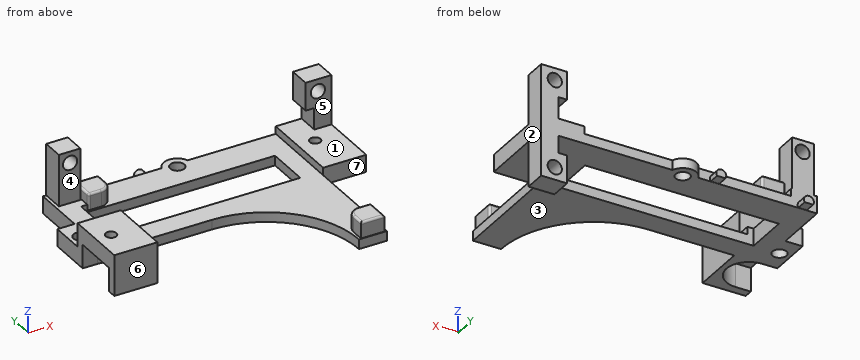
```python
from build123d import *

# Parameters (mm, degrees)
SKETCH021_R      = 1.65
EXTRUDE021_DEPTH = 5
EXTRUDE001_DEPTH = 4
FILLET003_R      = 0.5
BOX005_W         = 48
BOX005_H         = 47
BOX005_DEPTH     = 10
EXTRUDE037_DEPTH = 6
SKETCH038_W      = 10
SKETCH038_H      = 14.5
SKETCH038_R      = 1.25
EXTRUDE038_DEPTH = 4
SKETCH039_W      = 5
SKETCH039_H      = 16
SKETCH039_R      = 1.65
EXTRUDE039_DEPTH = 5
EXTRUDE040_DEPTH = 3
SKETCH020_R      = 1.65
SKETCH020_R_2    = 1.25
SKETCH020_W      = 45
SKETCH020_H      = 10
EXTRUDE036_DEPTH = 4


with BuildPart() as gpshold:
    # Sketch021 → Extrude021 (new body)
    with BuildSketch(Plane.XZ):
        Polygon((65, 28.5), (71, 28.5), (71, 2.5), (65, 2.5), (65, 9), (67, 9), (67, 22), (65, 22), align=None)
        with Locations((67.85, 25.7)):
            Circle(SKETCH021_R, mode=Mode.SUBTRACT)
        with Locations((67.85, 5.4)):
            Circle(SKETCH021_R, mode=Mode.SUBTRACT)
    extrude(amount=EXTRUDE021_DEPTH)


with BuildPart() as gpshold_1:
    # Extrude021 placement: moved
    add(gpshold.part.moved(Location((0, 78.75, 0))))


with BuildPart() as obj1:
    # Sketch001 → Extrude001 (new body)
    with BuildSketch(Plane.XY):
        with BuildLine():
            Line((19.03, 74.44), (19.03, 77.44))
            Line((19.03, 77.44), (13.53, 77.44))
            Line((13.53, 71.94), (13.53, 77.44))
            Line((16.53, 71.94), (13.53, 71.94))
            ThreePointArc((16.53, 71.94), (18.297767, 72.672233), (19.03, 74.44))
        make_face()
        with BuildLine():
            Line((60.53, 34.86), (55.03, 34.86))
            Line((55.03, 34.86), (55.03, 37.86))
            ThreePointArc((57.53, 40.36), (55.762233, 39.627767), (55.03, 37.86))
            Line((60.53, 40.36), (57.53, 40.36))
            Line((60.53, 34.86), (60.53, 40.36))
        make_face()
    extrude(amount=EXTRUDE001_DEPTH)


with BuildPart() as obj1_1:
    # Extrude001 placement: moved
    add(obj1.part.moved(Location((0, 0, 2))))

    # Fillet003
    fillet003_edges = [obj1_1.edges().sort_by_distance(p)[0] for p in [
        (57.78, 34.86, 6),
        (55.03, 36.36, 6),
        (55.762233, 39.627767, 6),
        (60.53, 40.36, 4),
        (59.03, 40.36, 6),
        (60.53, 37.61, 6),
        (18.297767, 72.672233, 6),
        (19.03, 77.44, 4),
        (19.03, 75.94, 6),
        (13.53, 77.44, 4),
        (16.28, 77.44, 6),
        (13.53, 71.94, 4),
        (13.53, 74.69, 6),
        (15.03, 71.94, 6),
    ]]
    fillet(fillet003_edges, radius=FILLET003_R)


with BuildPart() as obj1_2:
    # Fillet003 placement: moved
    add(obj1_1.part.moved(Location((0, 0, 13))))


with BuildPart() as obj2:
    # Box005 → Box005 (new body)
    with BuildSketch(Plane(origin=(13, 34, 15.25), x_dir=(1, 0, 0), z_dir=(0, 0, 1))):
        with Locations((24, 23.5)):
            Rectangle(BOX005_W, BOX005_H)
    extrude(amount=BOX005_DEPTH)


with BuildPart() as obj3:
    # Sketch037 → Extrude037 (new body)
    with BuildSketch(Plane.XY.offset(17)):
        with BuildLine():
            Line((3, 58.25), (13, 58.25))
            Line((13, 58.25), (13, 43.75))
            Line((13, 43.75), (3, 43.75))
            Line((3, 43.75), (3, 45.75))
            Line((3, 45.75), (6.5, 45.75))
            ThreePointArc((6.5, 45.75), (11.75, 51), (6.5, 56.25))
            Line((3, 56.25), (6.5, 56.25))
            Line((3, 58.25), (3, 56.25))
        make_face()
    extrude(amount=EXTRUDE037_DEPTH)


with BuildPart() as obj3_1:
    # Extrude037 placement: moved
    add(obj3.part.moved(Location((0, 0, -4))))


with BuildPart() as obj4:
    # Sketch038 → Extrude038 (new body)
    with BuildSketch(Plane.XY.offset(17)):
        with Locations((8, 51)):
            Rectangle(SKETCH038_W, SKETCH038_H)
        with Locations((6.5, 51)):
            Circle(SKETCH038_R, mode=Mode.SUBTRACT)
    extrude(amount=EXTRUDE038_DEPTH)


with BuildPart() as obj4_1:
    # Extrude038 placement: moved
    add(obj4.part.moved(Location((0, 0, 1.5))))


with BuildPart() as obj5:
    # Sketch039 → Extrude039 (new body)
    with BuildSketch(Plane.XZ.offset(-78.75)):
        with Locations((10.25, 21)):
            Rectangle(SKETCH039_W, SKETCH039_H)
        with Locations((10.35, 26.35)):
            Circle(SKETCH039_R, mode=Mode.SUBTRACT)
    extrude(amount=EXTRUDE039_DEPTH)


with BuildPart() as obj6:
    # Sketch040 → Extrude040 (new body)
    with BuildSketch(Plane.XZ.offset(-78.75)):
        with BuildLine():
            ThreePointArc((11.321071, 13.05), (10.34, 14.8), (9.358929, 13.05))
            Line((9.358929, 13.05), (11.321071, 13.05))
        make_face()
        with BuildLine():
            ThreePointArc((31.651071, 13.05), (30.67, 14.8), (29.688929, 13.05))
            Line((29.688929, 13.05), (31.651071, 13.05))
        make_face()
    extrude(amount=EXTRUDE040_DEPTH)


with BuildPart() as obj6_1:
    # Extrude040 placement: moved
    add(obj6.part.moved(Location((0, 2.5, 0))))


with BuildPart() as sensorhold005:
    # Sketch020 → Extrude036 (new body)
    with BuildSketch(Plane.XY):
        with BuildLine():
            Line((71, 78.75), (71, 60))
            Line((61, 60), (71, 60))
            Line((61, 34.75), (61, 60))
            Line((61, 34.75), (61, 60))
            Line((61, 34.75), (61, 60))
            Line((54.5, 34.75), (61, 34.75))
            ThreePointArc((54.5, 34.75), (48.202796, 49.952796), (33, 56.25))
            Line((3, 56.25), (33, 56.25))
            Line((3, 56.25), (3, 66.25))
            Line((3, 66.25), (7, 66.25))
            Line((7, 66.25), (7, 78.75))
            Line((7, 78.75), (34.55, 78.75))
            ThreePointArc((40.55, 78.75), (37.55, 80.878443), (34.55, 78.75))
            Line((40.55, 78.75), (71, 78.75))
        make_face()
        with Locations((5.55, 61.45)):
            Circle(SKETCH020_R, mode=Mode.SUBTRACT)
        with Locations((37.55, 77.7)):
            Circle(SKETCH020_R, mode=Mode.SUBTRACT)
        with Locations((65, 70)):
            Circle(SKETCH020_R_2, mode=Mode.SUBTRACT)
        with Locations((34.05, 66.45)):
            Rectangle(SKETCH020_W, SKETCH020_H, mode=Mode.SUBTRACT)
    extrude(amount=EXTRUDE036_DEPTH)


with BuildPart() as sensorhold005_1:
    # Extrude036 placement: moved
    add(sensorhold005.part.moved(Location((0, 0, 13))))

    # Fusion034: union obj3, obj4, obj5, obj6
    add(obj3_1.part)
    add(obj4_1.part)
    add(obj5.part)
    add(obj6_1.part)

    # Cut016: cut obj2
    add(obj2.part, mode=Mode.SUBTRACT)

    # Fusion035: union obj1
    add(obj1_2.part)

    # Fusion036: union gpsHold
    add(gpshold_1.part)


solid = sensorhold005_1.part
```
For this review, take the finished solid that the model builds, in its own axes (mm). Face numbers are marked on the shaded views. A direction names the side the tool comes from. Round coordinates to 2 decimals unless told otherwise and drop trailing zeros. Write each loop counter-clockwise with the first axis right and the second up, starting at its lowest first coordinate (ties: lowest second). Pieces come first, ordered by that corner, then holes. Notation, with made-up numbers: (56.5, 88.5) - (101.5, 88.5) arc R25 ccw to (101.5, 106.5) - close; hole circle Ø3 at (58.5, -20.75). An arc over 180 degrees is marked (long way). Write each question's results on one line, items separated by ' | '.
Item 1: For the marked faces 4, 5, 6 and 7, list the 3-axis set-ups (+Z, -Z, +X, -X, +Y, -Y) from which the entire face can be reached by the end or side of a thin tool; tool diameter is ignored.
Calculated:
face 4: +Z, -X | face 5: +Z, +X, -Y | face 6: +Z, -Z, -X, -Y | face 7: +Z, -Z, +X, -Y
Item 2: Take a section at B-B on y = 64. State the section outline as (x, z) points, then the cut area to 3 significant figures.
Calculated:
outline: (3, 13) - (11.55, 13) - (11.55, 17) - (3, 17) - close; (56.55, 13) - (71, 13) - (71, 17) - (61, 17) - (61, 15.25) - (56.55, 15.25) - close | area: 84.2 mm^2
Item 3: Take a section at D-D on y = 51. State the section outline as (x, z) points.
Calculated:
outline: (3, 18.5) - (5.25, 18.5) - (5.25, 22.5) - (3, 22.5) - close; (7.75, 18.5) - (11.75, 18.5) - (11.75, 13) - (13, 13) - (13, 22.5) - (7.75, 22.5) - close; (47.08, 13) - (61, 13) - (61, 15.25) - (47.08, 15.25) - close
Item 4: Take a section at A-A on x = 30.67. State the section outline as (y, z) points.
Calculated:
outline: (56.25, 13) - (61.45, 13) - (61.45, 15.25) - (56.25, 15.25) - close; (71.45, 13) - (78.75, 13) - (78.75, 13.05) - (81.25, 13.05) - (81.25, 14.8) - (78.75, 14.8) - (78.75, 15.25) - (71.45, 15.25) - close
Item 5: Take a section at C-C on x = 67.85. State the section outline as (y, z) points, then the cut area to 3 significant figures.
Calculated:
outline: (60, 13) - (73.75, 13) - (73.75, 7.05) - (78.75, 7.05) - (78.75, 24.05) - (73.75, 24.05) - (73.75, 17) - (60, 17) - close; (73.75, 2.5) - (78.75, 2.5) - (78.75, 3.75) - (73.75, 3.75) - close; (73.75, 27.35) - (78.75, 27.35) - (78.75, 28.5) - (73.75, 28.5) - close | area: 152 mm^2
Item 6: Draft analysis for pull direction X (two halves, no side actions). For the marked faces 1, 2 and 3, state which applies: pulls with the +X half, pulls with the -X half, needs draft (parallel to the pull), parting line crosses it, or undercut.
Calculated:
face 1: undercut | face 2: pulls with the +X half | face 3: needs draft
Item 7: To check wall thickness, follow line 1 along X through (y, z) = (70, 14.45); line 2 along Y through (x, z) = (37.55, 14.2); line 3 along X through (y, z) = (74, 16.75). State the ranges of each line that lie inside material, in increasing order. Write a range as from..to.
Calculated:
line 1: x = 7..11.55, 56.55..63.75, 66.25..71 | line 2: y = 55.76..61.45, 71.45..76.05, 79.35..80.88 | line 3: x = 7..13, 13.53..18.99, 61..71
Item 8: For pin 1 (4.5 mm diameter, centred on x = 6, y = 49.5, fed in from -Z); pin 2 (3 mm diameter, centred on y = 71, z = 14.5, fed in from -X); pin 3 (4 mm diameter, centred on x = 51.5, y = 45.5, fed in from -Z); pin 4 (8 mm diameter, centred on y = 58.5, z = 10, fed in from +X), all flat-tipped, find the tip position at first contact; note any pin that passes through.
Calculated:
pin 1: stops at z = 18.5 | pin 2: stops at x = 7 | pin 3: stops at z = 13 | pin 4: stops at x = 71
